```python
from build123d import *

# Parameters (mm, degrees)
PAD_DEPTH           = 400
SKETCH001_R         = 3
POCKET_DEPTH        = 4.5
SKETCH002_R         = 1.75
POCKET001_DEPTH     = 8.001
LINEARPATTERN_COUNT = 15
LINEARPATTERN_PITCH = 26.785714


with BuildPart() as part:
    # Sketch → Pad (new body)
    with BuildSketch(Plane.XZ):
        with BuildLine():
            Line((-5.5, 0), (5.5, 0))
            ThreePointArc((5.5, 0), (5.853553, 0.146447), (6, 0.5))
            Line((6, 0.5), (6, 4.5))
            ThreePointArc((6, 4.5), (5.853553, 4.853553), (5.5, 5))
            Line((5.5, 5), (4, 5))
            Line((4, 5), (4, 6))
            Line((4, 6), (5.5, 6))
            ThreePointArc((5.5, 6), (5.853553, 6.146447), (6, 6.5))
            Line((6, 6.5), (6, 7.5))
            ThreePointArc((6, 7.5), (5.853553, 7.853553), (5.5, 8))
            Line((-5.5, 8), (5.5, 8))
            ThreePointArc((-5.5, 8), (-5.853553, 7.853553), (-6, 7.5))
            Line((-6, 6.5), (-6, 7.5))
            ThreePointArc((-6, 6.5), (-5.853553, 6.146447), (-5.5, 6))
            Line((-4, 6), (-5.5, 6))
            Line((-4, 5), (-4, 6))
            Line((-5.5, 5), (-4, 5))
            ThreePointArc((-5.5, 5), (-5.853553, 4.853553), (-6, 4.5))
            Line((-6, 0.5), (-6, 4.5))
            ThreePointArc((-6, 0.5), (-5.853553, 0.146447), (-5.5, 0))
        make_face()
    extrude(amount=PAD_DEPTH)

    # Sketch001 (on Face12 of Pad) → Pocket (cut)
    with BuildSketch(Plane(origin=(0, 0, 8), x_dir=(-1, 0, 0), z_dir=(0, 0, 1))):
        with Locations((0, 10)):
            Circle(SKETCH001_R)
    pocket = extrude(amount=-POCKET_DEPTH, mode=Mode.SUBTRACT)

    # Sketch002 (on Face16 of Pocket) → Pocket001 (cut, through all)
    with BuildSketch(Plane(origin=(0, 0, 8), x_dir=(-1, 0, 0), z_dir=(0, 0, 1))):
        with Locations((0, 10)):
            Circle(SKETCH002_R)
    pocket001 = extrude(amount=-POCKET001_DEPTH, mode=Mode.SUBTRACT)

    # LinearPattern: Pocket, Pocket001 ×15
    with Locations(*[(0, -i * LINEARPATTERN_PITCH, 0) for i in range(1, LINEARPATTERN_COUNT)]):
        add(pocket, mode=Mode.SUBTRACT)
        add(pocket001, mode=Mode.SUBTRACT)


solid = part.part
```
For this review, take the finished solid that the model builds, in its own axes (mm). Round coordinates to 2 decimals unless told otherwise and drop trailing zeros. Write each loop counter-clockwise with the first axis right and the second up, starting at its lowest first coordinate (ties: lowest second). Pieces come first, ordered by that corner, then holes. Notation, with made-up numbers: (0, -25.5) - (13, -25.5) arc R16 ccw to (13, -21.5) - close; hole circle Ø5 at (-18, 71). An arc over 180 degrees is marked (long way). Write each question's results on one line, items separated by ' | '.
Item 1: Take a section at B-B on z = 2.25. Count the separate pieces of the cut face and the enclosed holes in it, then the cut area to 3 significant figures.
Calculated:
separate pieces: 1 | enclosed holes: 15 | area: 4,660 mm^2
Item 2: For pin 1 (4.5 mm diameter, centred on x = 0, y = -143.93, fed in from +Z), flat-tipped, find the tip position at first contact; note if it passes through.
Calculated:
pin 1: stops at z = 3.5
Item 3: Take a section at A-A on y = -341. State the section outline as (x, z) points.
Calculated:
outline: (-6, 0.5) arc R0.5 ccw to (-5.5, 0) - (5.5, 0) arc R0.5 ccw to (6, 0.5) - (6, 4.5) arc R0.5 ccw to (5.5, 5) - (4, 5) - (4, 6) - (5.5, 6) arc R0.5 ccw to (6, 6.5) - (6, 7.5) arc R0.5 ccw to (5.5, 8) - (-5.5, 8) arc R0.5 ccw to (-6, 7.5) - (-6, 6.5) arc R0.5 ccw to (-5.5, 6) - (-4, 6) - (-4, 5) - (-5.5, 5) arc R0.5 ccw to (-6, 4.5) - close
Item 4: To check wall thickness, follow line 1 along X through (y, z) = (-64, 2.25); line 2 along Z through (x, y) = (5, -146.5); line 3 along X through (y, z) = (-227, 5.5). State the ranges of each line that lie inside material, in increasing order. Write a range as from..to.
Calculated:
line 1: x = -6..-1.7, 1.7..6 | line 2: z = 0..5, 6..8 | line 3: x = -4..-1.28, 1.28..4
